Answer from the drawing. Dimensions are ordinates in mm from the lowest x, y and z of the part. A direction names the side the tool comes from. Round coordinates to 2 decimals unless told otherwise and drop trailing zeros. Loops run counter-clockwise (first coordinate to the right, second up) from the corner with the lowest first, then second, coordinate; pieces in that order, holes last. Notation, with made-up numbers: (15, 15.25) -> (58, 15.25) arc R13 ccw to (58, 19.25) -> close; hole circle Ø4 at (-17, 46.25). An arc over 180 degrees is marked (long way). One line per question, with ' | ' between items.
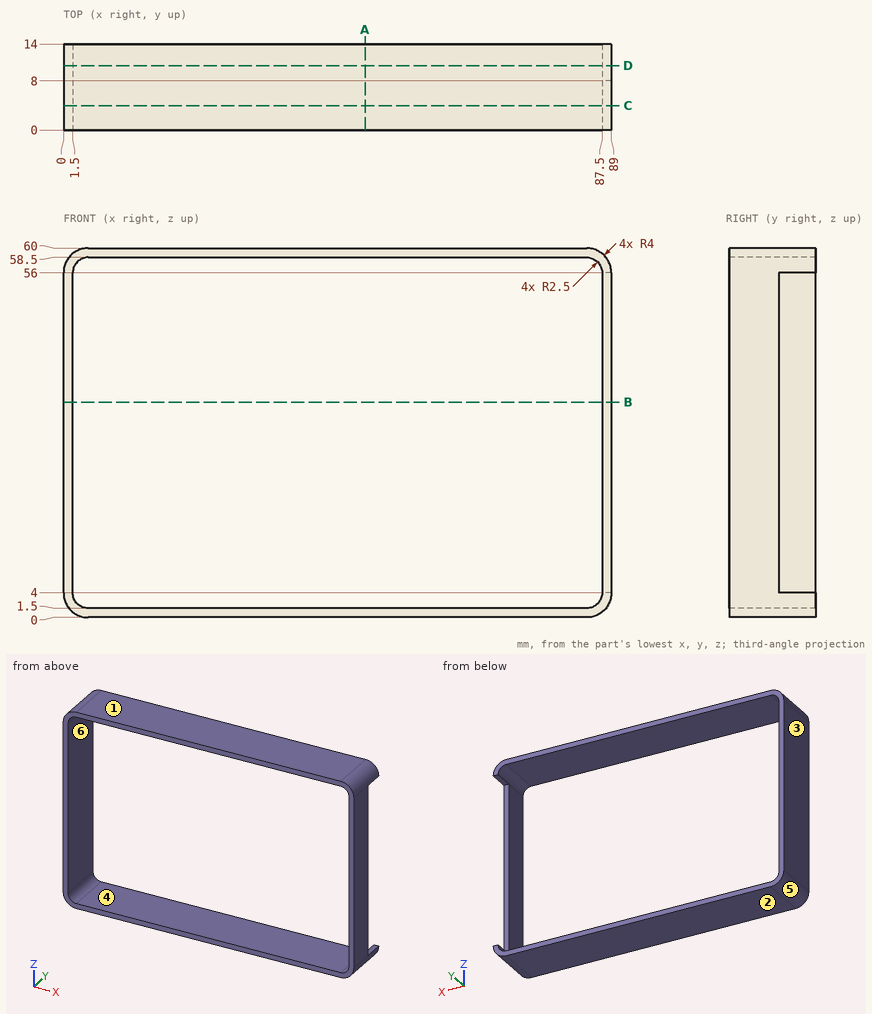
Q1. A cutting plane is placed at C-C on y = 4. Give the vertices of the cut face in (x, z).
Numbers:
outline: (0, 4) arc R4 ccw to (4, 0) -> (85, 0) arc R4 ccw to (89, 4) -> (89, 56) arc R4 ccw to (85, 60) -> (4, 60) arc R4 ccw to (0, 56) -> close; hole (1.5, 4) arc R2.5 ccw to (4, 1.5) -> (85, 1.5) arc R2.5 ccw to (87.5, 4) -> (87.5, 56) arc R2.5 ccw to (85, 58.5) -> (4, 58.5) arc R2.5 ccw to (1.5, 56) -> close
Q2. A cutting plane is placed at D-D on y = 10.5. Give the vertices of the cut face in (x, z), plus the area to 3 significant figures.
Numbers:
outline: (0, 4) arc R4 ccw to (4, 0) -> (85, 0) arc R4 ccw to (89, 4) -> (87.5, 4) arc R2.5 cw to (85, 1.5) -> (4, 1.5) arc R2.5 cw to (1.5, 4) -> (1.5, 56) arc R2.5 cw to (4, 58.5) -> (85, 58.5) arc R2.5 cw to (87.5, 56) -> (89, 56) arc R4 ccw to (85, 60) -> (4, 60) arc R4 ccw to (0, 56) -> close | area: 352 mm^2
Q3. A cutting plane is placed at B-B on z = 35. Give the vertices of the cut face in (x, y), plus the area to 3 significant figures.
Numbers:
outline: (0, 0) -> (1.5, 0) -> (1.5, 14) -> (0, 14) -> close; (87.5, 0) -> (89, 0) -> (89, 8) -> (87.5, 8) -> close | area: 33.0 mm^2
Q4. Given pin 1 Ø1.6 at (x, z) = (88, 21) entering from +Y; pin 2 Ø0.8 at (x, y) = (88.5, 10) entering from +Z; pin 3 Ø0.8 at (x, y) = (88, 10.5) entering from -Z, each flat-ended and moving along its own axis, determine where each tip first touches the part or whether it passes through.
Numbers:
pin 1: y = 8 | pin 2: z = 58.53 | pin 3: z = 0.96
Q5. A cutting plane is placed at A-A on x = 49. Give the vertices of the cut face in (y, z).
Numbers:
outline: (0, 0) -> (14, 0) -> (14, 1.5) -> (0, 1.5) -> close; (0, 58.5) -> (14, 58.5) -> (14, 60) -> (0, 60) -> close
Q6. For the marked faces 5 and 6, determine the directions among +Z, -Z, +X, -X, +Y, -Y from which every point of the face is accessible in a straight line to the end or side of a thin tool.
Numbers:
face 5: -Z, -X, +Y, -Y | face 6: +Y, -Y
Q7. For a pull along Z with two mould halves and no side action, classify the marked faces 1, 2, 3 and 4 as pulls with the +Z half, pulls with the -Z half, needs draft (parallel to the pull), parting line crosses it, or undercut.
Numbers:
face 1: pulls with the +Z half | face 2: pulls with the -Z half | face 3: needs draft | face 4: undercut
Q8. Find the intervals of material crossed by line 1 (Z direction, x = 18, y = 6.25); line 2 (X direction, y = 1.75, z = 25.5); line 3 (X direction, y = 13.25, z = 19), in increasing order. Write a range as from..to.
Numbers:
line 1: 0..1.5, 58.5..60 | line 2: 0..1.5, 87.5..89 | line 3: 0..1.5
